```python
from build123d import *

# Parameters (mm, degrees)
SKETCH3_W                = 40
SKETCH3_H                = 40
SKETCH3_W_2              = 34
SKETCH3_H_2              = 34
BOSS_EXTRUDE2_REACH      = 64.147
SKETCH7_W                = 16
SKETCH7_H                = 28
BOSS_EXTRUDE5_DEPTH      = 1
BOSS_EXTRUDE5_DEPTH_BACK = 5
SKETCH8_W                = 13
SKETCH8_H                = 40
CHAMFER1_SIZE            = 6
CHAMFER2_SIZE            = 4
SKETCH9_W                = 14
SKETCH9_H                = 3
CUT_EXTRUDE1_DEPTH       = 16
SKETCH10_W               = 12
SKETCH10_H               = 24
CUT_EXTRUDE2_DEPTH       = 72.149717806
SKETCH11_W               = 15
SKETCH11_H               = 40
BOSS_EXTRUDE6_DEPTH      = 7
CUT_EXTRUDE3_DEPTH       = 66.163504693
CUT_EXTRUDE4_REACH       = 60.927
SKETCH13_W               = 12
SKETCH13_H               = 3.5
SKETCH15_W               = 4.5
SKETCH15_H               = 4.5
BOSS_EXTRUDE7_DEPTH      = 5
SKETCH14_R               = 1.5
CUT_EXTRUDE5_DEPTH       = 8
CHAMFER3_SIZE            = 14
CHAMFER7_SIZE            = 3
CHAMFER4_SIZE            = 14
CHAMFER5_SIZE            = 2
CHAMFER9_SIZE            = 2
CHAMFER10_SIZE           = 2.121320344
CHAMFER10_SIZE_2         = 1.5
CHAMFER11_SIZE           = 10
CHAMFER12_SIZE           = 2


# Some blends are built 0.0001 mm under size
with BuildPart() as part:
    # Sweep1: sweep along a path in Sketch2
    with BuildLine(Plane.XY) as sweep1_path:
        Line((0, 0), (-5, 0))
        ThreePointArc((-5, 0), (-20.718824406, 2.771652848), (-34.541726603, 10.752309152))
        Line((-34.541726603, 10.752309152), (-38.371948819, 13.966247201))
    # Sketch3 → Sweep1 (sweep)
    with BuildSketch(Plane(origin=(0, 0, 0), x_dir=(0, 0, -1), z_dir=(1, 0, 0))):
        with Locations((0, 20)):
            Rectangle(SKETCH3_W, SKETCH3_H)
        with Locations((0, 20)):
            Rectangle(SKETCH3_W_2, SKETCH3_H_2, mode=Mode.SUBTRACT)
    sweep(path=sweep1_path.line)

    # Boss-Extrude2: up to this face of the body (flat: up to its plane)
    boss_extrude2_end = Plane(part.part.faces().sort_by_distance((-2.5, 40, 0))[0])
    # Sketch7 → Boss-Extrude2 (add, up to the picked face)
    with BuildSketch(Plane(origin=(0, 0, 0), x_dir=(1, 0, 0), z_dir=(0, 1, 0)), mode=Mode.PRIVATE) as boss_extrude2_sk1:
        with Locations((8, -6)):
            Rectangle(SKETCH7_W, SKETCH7_H)
    boss_extrude2_tool1 = split(extrude(boss_extrude2_sk1.sketch, amount=BOSS_EXTRUDE2_REACH, mode=Mode.PRIVATE), bisect_by=boss_extrude2_end, keep=Keep.BOTH, mode=Mode.PRIVATE)
    add(boss_extrude2_tool1.solids().sort_by(Axis((8, 0, 6), (0, 1, 0)))[0])

    # Sketch8 → Boss-Extrude5 (add, two sides: drawn at the far end of the back side and taken through both)
    with BuildSketch(Plane(origin=(0, 0, 0), x_dir=(0, 0, -1), z_dir=(1, 0, 0)).offset(-BOSS_EXTRUDE5_DEPTH_BACK)):
        with Locations((13.5, 20)):
            Rectangle(SKETCH8_W, SKETCH8_H)
    extrude(amount=BOSS_EXTRUDE5_DEPTH + BOSS_EXTRUDE5_DEPTH_BACK)

    # Chamfer1
    chamfer1_edges = [part.edges().sort_by_distance(p)[0] for p in [
        (-5, 20, -17),
    ]]
    chamfer(chamfer1_edges, length=CHAMFER1_SIZE)

    # Chamfer2
    chamfer2_edges = [part.edges().sort_by_distance(p)[0] for p in [
        (-5, 20, -7),
    ]]
    chamfer(chamfer2_edges, length=CHAMFER2_SIZE - 0.0001)  # a hair under: the kernel refuses the full size

    # Sketch9 → Cut-Extrude1 (cut)
    with BuildSketch(Plane(origin=(16, 0, 0), x_dir=(0, 0, -1), z_dir=(1, 0, 0))):
        with Locations((0, 2.5)):
            Rectangle(SKETCH9_W, SKETCH9_H)
    extrude(amount=-CUT_EXTRUDE1_DEPTH, mode=Mode.SUBTRACT)

    # Sketch10 → Cut-Extrude2 (cut, through all)
    with BuildSketch(Plane.XY.offset(20)):
        with Locations((10, 28)):
            Rectangle(SKETCH10_W, SKETCH10_H)
    extrude(amount=-CUT_EXTRUDE2_DEPTH, mode=Mode.SUBTRACT)

    # Sketch11 → Boss-Extrude6 (add)
    with BuildSketch(Plane(origin=(0, 0, -8), x_dir=(-1, 0, 0), z_dir=(0, 0, -1))):
        with Locations((-8.5, 20)):
            Rectangle(SKETCH11_W, SKETCH11_H)
    extrude(amount=BOSS_EXTRUDE6_DEPTH)

    # Sketch12 → Cut-Extrude3 (cut, through all)
    with BuildSketch(Plane.XY.offset(-8)):
        with BuildLine():
            Line((11.75, 36), (11.75, 20))
            ThreePointArc((11.75, 20), (10, 18.25), (8.25, 20))
            Line((8.25, 20), (8.25, 36))
            ThreePointArc((8.25, 36), (10, 37.75), (11.75, 36))
        make_face()
    extrude(amount=-CUT_EXTRUDE3_DEPTH, mode=Mode.SUBTRACT)

    # Cut-Extrude4: up to this face of the body (flat: up to its plane)
    cut_extrude4_end = Plane(part.part.faces().sort_by_distance((10, 16, 6))[0])
    # Sketch13 → Cut-Extrude4 (cut, up to the picked face)
    with BuildSketch(Plane(origin=(0, 40, 0), x_dir=(1, 0, 0), z_dir=(0, 1, 0)), mode=Mode.PRIVATE) as cut_extrude4_sk1:
        with Locations((10, 9.75)):
            Rectangle(SKETCH13_W, SKETCH13_H)
    cut_extrude4_tool1 = split(extrude(cut_extrude4_sk1.sketch, amount=-CUT_EXTRUDE4_REACH, mode=Mode.PRIVATE), bisect_by=cut_extrude4_end, keep=Keep.BOTH, mode=Mode.PRIVATE)
    add(cut_extrude4_tool1.solids().sort_by(Axis((10, 40, -9.75), (0, -1, 0)))[0], mode=Mode.SUBTRACT)

    # Sketch15 → Boss-Extrude7 (add)
    with BuildSketch(Plane(origin=(-29.394618164, 24.66501326, 0), x_dir=(0, 0, 1), z_dir=(-0.7660444431189811, 0.6427876096865356, 0))):
        with Locations((-14.75, 20.783752799)):
            Rectangle(SKETCH15_W, SKETCH15_H)
        with Locations((14.75, 20.783752799)):
            Rectangle(SKETCH15_W, SKETCH15_H)
        with Locations((-14.75, -8.716247201)):
            Rectangle(SKETCH15_W, SKETCH15_H)
        with Locations((14.75, -8.716247201)):
            Rectangle(SKETCH15_W, SKETCH15_H)
    extrude(amount=-BOSS_EXTRUDE7_DEPTH)

    # Sketch14 → Cut-Extrude5 (cut)
    with BuildSketch(Plane(origin=(-29.394618164, 24.66501326, 0), x_dir=(0, 0, 1), z_dir=(-0.7660444431189811, 0.6427876096865356, 0))):
        with Locations(Location((-16, 22.033752799, 0), (0, 0, 270))):
            Circle(SKETCH14_R)
        with Locations(Location((16, 22.033752799, 0), (0, 0, 270))):
            Circle(SKETCH14_R)
        with Locations(Location((-16, -9.966247201, 0), (0, 0, 270))):
            Circle(SKETCH14_R)
        with Locations(Location((16, -9.966247201, 0), (0, 0, 270))):
            Circle(SKETCH14_R)
    extrude(amount=-CUT_EXTRUDE5_DEPTH, mode=Mode.SUBTRACT)

    # Chamfer3
    chamfer3_edges = [part.edges().sort_by_distance(p)[0] for p in [
        (0, 4, 0),
    ]]
    chamfer(chamfer3_edges, length=CHAMFER3_SIZE)

    # Chamfer7
    # the kernel refuses this chamfer: 3 mm, written as the material it takes off along each edge
    with BuildSketch(Plane(origin=(16, 0, 27.715048964), x_dir=(0.027495876610586778, 0.9996219169112968, 0), z_dir=(0, 0, -1))) as chamfer7_piece_1:
        Polygon((CHAMFER7_SIZE * 0.999621916911, -CHAMFER7_SIZE * 0.0274958766106), (-CHAMFER7_SIZE * 0.0274958766106, -CHAMFER7_SIZE * 0.999621916911), (0, 0), align=None)
    extrude(amount=50.430097928, mode=Mode.SUBTRACT)

    # Chamfer4
    # the kernel refuses this chamfer: 14 mm, written as the material it takes off along each edge
    with BuildSketch(Plane(origin=(0, 54.003561832, 7), x_dir=(-0.027495876610586376, 0, 0.9996219169112968), z_dir=(0, -1, 0))) as chamfer4_piece_1_section:
        Polygon((CHAMFER4_SIZE * 0.999621916911, -CHAMFER4_SIZE * 0.0274958766106), (-CHAMFER4_SIZE * 0.0274958766106, -CHAMFER4_SIZE * 0.999621916911), (0, 0), align=None)
    chamfer4_piece_1 = extrude(amount=51.003561832, mode=Mode.PRIVATE)
    chamfer4_piece_1 = split(chamfer4_piece_1, bisect_by=Plane(origin=(0.666666667, 16.666666667, 17), z_dir=(0, 0, -1)), keep=Keep.TOP, mode=Mode.PRIVATE)
    chamfer4_piece_1 = split(chamfer4_piece_1, bisect_by=Plane(origin=(1, 17, 12), z_dir=(-0.7071067811865476, -0.7071067811865476, 0)), keep=Keep.TOP, mode=Mode.PRIVATE)
    add(chamfer4_piece_1, mode=Mode.SUBTRACT)

    # Chamfer5
    chamfer5_edges = [part.edges().sort_by_distance(p)[0] for p in [
        (0, 3, 0),
    ]]
    chamfer(chamfer5_edges, length=CHAMFER5_SIZE - 0.0001)  # a hair under: the kernel refuses the full size

    # Chamfer9
    chamfer9_edges = [part.edges().sort_by_distance(p)[0] for p in [
        (4, 16, 4.25),
        (4, 40, 4.25),
        (16, 40, -13.25),
    ]]
    chamfer(chamfer9_edges, length=CHAMFER9_SIZE)

    # Chamfer10
    # the kernel refuses this chamfer: 2.121320344, 1.5 mm, written as the material it takes off along each edge
    with BuildSketch(Plane(origin=(14, 1, -7), x_dir=(-0.9996219169112964, 0.02749587661059746, 0), z_dir=(0, 0, 1))) as chamfer10_piece_1:
        Polygon((CHAMFER10_SIZE * 0.999621916703, CHAMFER10_SIZE * 0.0274958766049), (CHAMFER10_SIZE_2 * 0.687396915265, CHAMFER10_SIZE_2 * 0.726281956876), (0, 0), align=None)
    extrude(amount=14, mode=Mode.SUBTRACT)

    # Chamfer11
    chamfer11_edges = [part.edges().sort_by_distance(p)[0] for p in [
        (16, 9.5, 20),
    ]]
    chamfer(chamfer11_edges, length=CHAMFER11_SIZE)

    # Chamfer12
    chamfer12_edges = [part.edges().sort_by_distance(p)[0] for p in [
        (-10.745333323, 43.001055901, -20),
        (-7.038018673, 40.359357679, -20),
        (-2, 40, -20),
        (-36.456837711, 12.359278177, -20),
        (-20.718824406, 2.771652848, -20),
        (-2, 0, -20),
        (-36.456837711, 12.359278177, 20),
        (-20.718824406, 2.771652848, 20),
        (0.5, 0, 20),
        (-10.745333323, 43.001055901, 20),
        (-7.038018673, 40.359357679, 20),
        (-1.5, 40, 20),
        (-31.635930638, 18.1046115, 12.5),
        (-15.566240396, 37.255722578, 12.5),
        (-15.566240396, 37.255722578, -12.5),
        (-31.635930638, 18.1046115, -12.5),
    ]]
    chamfer(chamfer12_edges, length=CHAMFER12_SIZE)


solid = part.part
```
Input: part model. Units: mm. Frame: model coordinates. A direction names the side the tool comes from. Coordinates: 2 decimals unless noted, no trailing zeros. Write each loop counter-clockwise with the first axis right and the second up, starting at its lowest first coordinate (ties: lowest second). Pieces come first, ordered by that corner, then holes.
1) Material intervals for line 1 along Y through (x, z) = (5, -6.5); line 2 along Y through (x, z) = (-1, 7.5); line 3 along X through (y, z) = (23, 11.5), sorted ascending.
2) Pin query (flat end, axial travel): pin 1 Ø5 at (x, z) = (10, 1) entering from +Y; pin 2 Ø2 at (y, z) = (37.5, 11) entering from -X; pin 3 Ø5 at (y, z) = (17.5, -3) entering from -X. Return the tip coordinate at first contact, or that it passes through.
3) Set-up query: faces 1 (the flat face through (11.75, 28, -13)), 2 (the flat face through (3, 39, 4)), 3 (the flat face through (7, 2, 7)). Return all of +Z, -Z, +X, -X, +Y, -Y with unobstructed straight access to the full face (end or side cutting, diameter ignored); none if empty.
4) Section A-A on x = 10. Output: boundary loops of the cut face in (y, z).
5) Mould query, pull axis Z, two halves, no side actions, for faces 4 (the flat face through (-36.48, 12.38, 0.25)), 5 (the flat face through (-2, 39, -19)), 6 (the flat face through (-30.35, 11.08, -16.64)). Classes: pulls with the +Z half, pulls with the -Z half, needs draft (parallel to the pull), parting line crosses it, or undercut.
6) Section D-D on z = 11. Output: boundary loops of the cut face in (x, y).
Check result:
1. line 1: y = 0 to 1, 13 to 17
1. line 2: y = 0 to 3, 37 to 40
1. line 3: x = 0 to 4
2. pin 1: stops at y = 16
2. pin 2: stops at x = -9.96
2. pin 3: stops at x = -37.5
3. face 1: +Z, -Z
3. face 2: +Z, +X, +Y
3. face 3: +X
4. outline: (0, -15) - (18.25, -15) - (18.25, -11.5) - (16, -11.5) - (16, 16) - (0, 16) - close; (37.75, -15) - (40, -15) - (40, -11.5) - (37.75, -11.5) - close; hole (1, -7) - (8, -7) - (8, 11) - (3, 11) - (3, 7) - (1, 7) - close
5. face 4: needs draft
5. face 5: pulls with the -Z half
5. face 6: undercut
6. outline: (-38.37, 13.97) - (-34.54, 10.75) arc R45.96 ccw to (-5, 0) - (13, 0) - (15, 2) - (15, 16) - (6, 16) - (4, 18) - (4, 38) - (2, 40) - (-5, 40) arc R5.96 cw to (-8.83, 41.39) - (-12.66, 44.61) - (-14.59, 42.31) - (-10.76, 39.1) arc R8.96 ccw to (-5, 37) - (0, 37) - (0, 18) - (10, 8) - (10, 3) - (-5, 3) arc R42.96 cw to (-32.61, 13.05) - (-36.44, 16.26) - close
